Geometry: see drawing. Coordinates: mm, zero at the bounding-box minimum. Give positions to 0.01 mm unless a question says otherwise; leave off trailing zeros. Write each loop counter-clockwise with the first axis right and the second up, starting at its lowest first coordinate (ties: lowest second). Pieces come first, ordered by that corner, then holes.
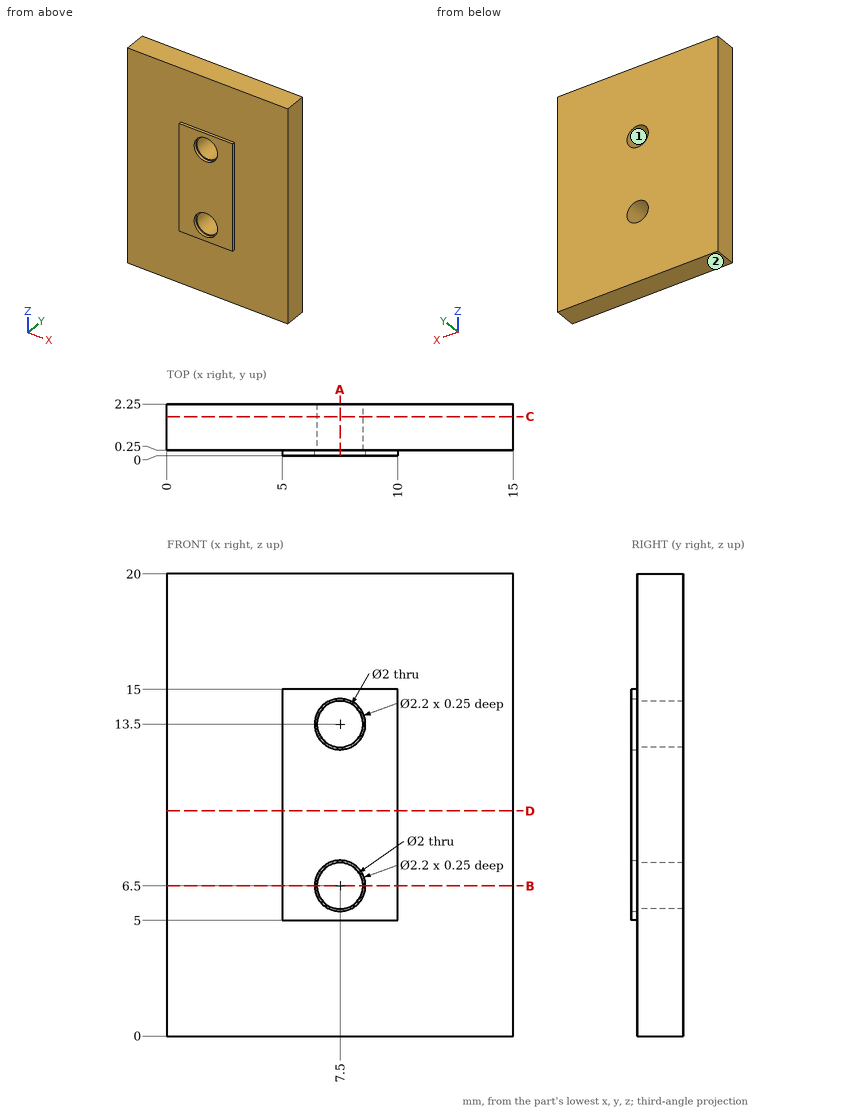
1. Pin query (flat end, axial travel): P1, Ø2.5, axis at x = 7.5, z = 6.5, coming from the -Y side; P2, Ø1.1, axis at x = 7.5, z = 7, coming from the -Y side. Return the tip coordinate at first contact, or that it passes through.
2. Section query B-B (z = 6.5). Return loops of the section in (x, y), plus the area to 3 significant figures.
3. Section query A-A (x = 7.5). Return loops of the section in (y, z).
4. Pull-direction query (X, two-part tool) for the marked faces 1 and 2; classes: pulls with the +X half, pulls with the -X half, needs draft (parallel to the pull), parting line crosses it, or undercut.
5. Section query C-C (y = 1.7). Return loops of the section in (x, z).
6. Line query: probe 1 along Z at (x, y) = (7.5, 1.7); probe 2 along Z at (x, y) = (7.5, 0.15); probe 3 along Y at (x, z) = (4, 7.75). Output: solid intervals per line, ascending.
7. Section query D-D (z = 9.75). Return loops of the section in (x, y), plus the area to 4 significant figures.
The answers:
1. P1: stops at y = 0
1. P2: stops at y = 0.25
2. outline: (0, 0.25) - (5, 0.25) - (5, 0) - (6.4, 0) - (6.4, 0.25) - (6.5, 0.25) - (6.5, 2.25) - (0, 2.25) - close; (8.5, 0.25) - (8.6, 0.25) - (8.6, 0) - (10, 0) - (10, 0.25) - (15, 0.25) - (15, 2.25) - (8.5, 2.25) - close
2. area: 26.7 mm2
3. outline: (0, 5) - (0.25, 5) - (0.25, 0) - (2.25, 0) - (2.25, 5.5) - (0.25, 5.5) - (0.25, 5.4) - (0, 5.4) - close; (0, 7.6) - (0.25, 7.6) - (0.25, 7.5) - (2.25, 7.5) - (2.25, 12.5) - (0.25, 12.5) - (0.25, 12.4) - (0, 12.4) - close; (0, 14.6) - (0.25, 14.6) - (0.25, 14.5) - (2.25, 14.5) - (2.25, 20) - (0.25, 20) - (0.25, 15) - (0, 15) - close
4. face 1: undercut
4. face 2: needs draft
5. outline: (0, 0) - (15, 0) - (15, 20) - (0, 20) - close; hole circle Ø2 at (7.5, 6.5); hole circle Ø2 at (7.5, 13.5)
6. probe 1: z = 0 to 5.5, 7.5 to 12.5, 14.5 to 20
6. probe 2: z = 5 to 5.4, 7.6 to 12.4, 14.6 to 15
6. probe 3: y = 0.25 to 2.25
7. outline: (0, 0.25) - (5, 0.25) - (5, 0) - (10, 0) - (10, 0.25) - (15, 0.25) - (15, 2.25) - (0, 2.25) - close
7. area: 31.25 mm2
